The model under review builds one solid part; all positions refer to its coordinate system, in mm. A direction names the side the tool comes from. Coordinates: 2 decimals unless noted, no trailing zeros. Write each loop counter-clockwise with the first axis right and the second up, starting at its lowest first coordinate (ties: lowest second). Pieces come first, ordered by that corner, then holes.
1) For P1, Ø2, axis at x = 49.5, z = 4.5, coming from the +Y side; P2, Ø2.5, axis at x = -60.5, y = 9, coming from the +Z side; P3, Ø6, axis at y = 1, z = 10, coming from the +X side; P4, Ø2.5, axis at x = 48.36, y = -15.34, coming from the +Z side, all flat-tipped, find the tip position at first contact; note any pin that passes through.
2) For line 1 (Y direction, x = 28.5, z = 12); line 2 (X direction, y = -11, z = 14.75); line 3 (X direction, y = 8, z = 3.75), list the stretches that pass through material, from the lowest coordinate up.
3) Add section A-A, the plane y = 10. State the section outline as (x, z) points.
4) Machinability: for faces 1 (the flat face through (-59.6, 13.2, 5)), 2 (the flat face through (50.36, -12, 7)), 3 (the flat face through (-58.84, -1, 6)), 4 (the flat face through (49, -8.341, 7)), 5 (the flat face through (-11.3, -17.4, 16)), which of the approach directions +Z, -Z, +X, -X, +Y, -Y give a long, thin tool a straight path to every point of the face, cutting with its end or side? Answer none if there is none.
5) Add section C-C, the plane z = 10.5. State the section outline as (x, y) points.
6) Add section B-B, the plane x = 17.5. State the section outline as (y, z) points, then the cut area to 3 significant figures.
Autodesk Inventor part; units mm, degrees
ref_plane "YZ Plane" through (0, 0, 0) normal (1, 0, 0) x (0, 1, 0)
ref_plane "XZ Plane" through (0, 0, 0) normal (0, 1, 0) x (-1, 0, 0)
ref_plane "XY Plane" through (0, 0, 0) normal (0, 0, 1) x (1, 0, 0)
sketch "Sketch1" plane through (0, 0, 0) normal (0, 0, 1) x (1, 0, 0)
  line L0 (-58.8402, 23.8593) -> (45.1598, 23.8593)
  line L1 (45.1598, 23.8593) -> (45.1598, -17.1407)
  line L2 (45.1598, -17.1407) -> (-58.8402, -17.1407)
  line L3 (-58.8402, -17.1407) -> (-58.8402, 23.8593)
  line L4 (-60.0402, 25.0593) -> (46.3598, 25.0593)
  line L5 (46.3598, 25.0593) -> (46.3598, -18.3407)
  line L6 (46.3598, -18.3407) -> (-60.0402, -18.3407)
  line L7 (-60.0402, -18.3407) -> (-60.0402, 25.0593)
  point P0 (0, 0)
  dimension "d0" = 104
  dimension "d1" = 41
  dimension "d2" = 1.2
  dimension "d3" = 1.2
  dimension "d4" = 1.2
  dimension "d5" = 1.2
extrude "Extrusion1" add sketch "Sketch1" along normal blind 16
sketch "Sketch2" plane through (0, 0, 0) normal (0, 0, -1) x (-1, 0, 0)
  line L0 (-46.3598, 25.0593) -> (60.0402, 25.0593)
  line L1 (60.0402, 25.0593) -> (60.0402, -18.3407)
  line L2 (60.0402, -18.3407) -> (-46.3598, -18.3407)
  line L3 (-46.3598, -18.3407) -> (-46.3598, 25.0593)
  point P0 (0, 0)
extrude "Extrusion2" add sketch "Sketch2" along normal blind 2
sketch "Sketch3" plane through (0, 0, 16) normal (0, 0, 1) x (1, 0, 0)
  line L0 (-60.0402, 25.0593) -> (-60.0402, -18.3407)
  line L1 (-58.8402, 23.8593) -> (-60.0402, 23.8593)
  line L2 (-60.0402, 23.8593) -> (-60.0402, 3.8593)
  line L3 (-60.0402, 3.8593) -> (-58.8402, 3.8593)
  line L4 (-58.8402, 3.8593) -> (-58.8402, 23.8593)
  point P0 (0, 0)
  dimension "d10" = 20
extrude "Extrusion3" cut sketch "Sketch3" against normal blind 11
sketch "Sketch4" plane through (0, 0, 16) normal (0, 0, 1) x (1, 0, 0)
  line L0 (-60.0402, -18.3407) -> (-64.0402, -18.3407)
  line L1 (-64.0402, -18.3407) -> (-64.0402, 3.8593)
  line L2 (-64.0402, 3.8593) -> (-60.0402, 3.8593)
  line L3 (-60.0402, 3.8593) -> (-60.0402, -18.3407)
  line L4 (-60.0402, 23.8593) -> (45.1598, 23.8593)
  line L5 (46.3598, 25.0593) -> (50.3598, 25.0593)
  line L6 (50.3598, 25.0593) -> (50.3598, 15.0593)
  line L7 (50.3598, 15.0593) -> (46.3598, 15.0593)
  line L8 (46.3598, 15.0593) -> (46.3598, 25.0593)
  line L9 (46.3598, -18.3407) -> (50.3598, -18.3407)
  line L10 (50.3598, -18.3407) -> (50.3598, -8.3407)
  line L11 (50.3598, -8.3407) -> (46.3598, -8.3407)
  line L12 (46.3598, -8.3407) -> (46.3598, -18.3407)
  point P0 (0, 0)
  dimension "d13" = 4
  dimension "d14" = 20
  dimension "d15" = 4
  dimension "d16" = 10
  dimension "d17" = 4
  dimension "d18" = 10
extrude "Extrusion4" add sketch "Sketch4" against normal blind 18
chamfer "Chamfer1" distance 2 angle 45 1 edges at (-60.0402, 3.8593, 1.5)
chamfer "Chamfer2" distance 2 angle 45 2 edges at (46.3598, 15.0593, 7) (46.3598, -8.3407, 7)
sketch "Sketch5" plane through (0, 0, 16) normal (0, 0, 1) x (1, 0, 0)
  line L0 (-60.0402, 25.0593) -> (50.3598, 25.0593)
  line L1 (50.3598, 25.0593) -> (50.3598, 15.0593)
  line L2 (50.3598, -18.3407) -> (50.3598, -8.3407)
  line L3 (50.3598, -18.3407) -> (-64.0402, -18.3407)
  line L4 (-64.0402, -18.3407) -> (-64.0402, 3.8593)
  point P0 (0, 0)
  point P1 (-62.0402, -15.3407)
  point P2 (48.3598, -15.3407)
  point P3 (48.3598, 22.0593)
  dimension "d27" = 3
  dimension "d28" = 2
  dimension "d29" = 2
  dimension "d30" = 3
  dimension "d31" = 3
  dimension "d32" = 2
  dimension "d33" = 110.4
  dimension "d34" = 37.4
hole "Hole1" at (-62.0402, -15.3407, 16) at (48.3598, -15.3407, 16) at (48.3598, 22.0593, 16) direction (0, 0, -1) diameter 2 depth 8 tip angle 118
chamfer "Chamfer3" distance 2 angle 45 3 edges at (50.3598, 25.0593, 7) (50.3598, -18.3407, 7) (-64.0402, -18.3407, 7)
properties part number "main body"
Geometry results:
1. P1: stops at y = 24.92
1. P2: stops at z = 5
1. P3: stops at x = 46.36
1. P4: stops at z = 16
2. line 1: y = -18.34 to -17.14, 23.86 to 25.06
2. line 2: x = -64.04 to -58.84, 45.16 to 50.36
2. line 3: x = -60.04 to -58.84, 45.16 to 46.36
3. outline: (-60.04, -2) - (46.36, -2) - (46.36, 16) - (45.16, 16) - (45.16, 0) - (-58.84, 0) - (-58.84, 5) - (-60.04, 5) - close
4. face 1: +Z, -X
4. face 2: +Z, -Z, +X, +Y, -Y
4. face 3: +Z
4. face 4: +Z, -Z, +X
4. face 5: +Z, +X, -X, +Y, -Y
5. outline: (-64.04, -16.34) - (-62.04, -18.34) - (48.36, -18.34) - (50.36, -16.34) - (50.36, -8.34) - (48.36, -8.34) - (46.36, -6.34) - (46.36, 13.06) - (48.36, 15.06) - (50.36, 15.06) - (50.36, 23.06) - (48.36, 25.06) - (-60.04, 25.06) - (-60.04, 23.86) - (45.16, 23.86) - (45.16, -17.14) - (-58.84, -17.14) - (-58.84, 3.86) - (-64.04, 3.86) - close; hole circle Ø2 at (-62.04, -15.34); hole circle Ø2 at (48.36, -15.34); hole circle Ø2 at (48.36, 22.06)
6. outline: (-18.34, -2) - (25.06, -2) - (25.06, 16) - (23.86, 16) - (23.86, 0) - (-17.14, 0) - (-17.14, 16) - (-18.34, 16) - close
6. area: 125 mm2
